Autodesk Inventor part; units mm, degrees
ref_plane "Work Plane1" through (0, 0, 1.25) normal (0, 0, 1) x (1, 0, 0)
ref_plane "YZ Plane" through (0, 0, 0) normal (1, 0, 0) x (0, 1, 0)
ref_plane "XZ Plane" through (0, 0, 0) normal (0, 1, 0) x (-1, 0, 0)
sketch "Sketch1" plane through (0, 0, 0) normal (0, 0, 1) x (1, 0, 0)
  circle A0 centre (0, 0) radius 5.5
  dimension "d0" = 11
extrude "Extrusion1" add sketch "Sketch1" along normal blind 2.5
hole "Hole1" at (0, 0, 2.5) direction (0, 0, -1) diameter 7 end through all
sketch "Sketch2" plane through (0, 0, 2.5) normal (0, 0, 1) x (1, 0, 0)
  circle A0 centre (0, 0) radius 5
  circle A1 centre (0, 0) radius 4
  dimension "d12" = 10
  dimension "d13" = 8
extrude "Extrusion2" cut sketch "Sketch2" against normal blind 0.5
ref_plane "Work Plane1" through (0, 0, 1.25) normal (0, 0, 1) x (1, 0, 0)
mirror "Mirror1" about plane through (0, 0, 1.25) normal (0, 0, 1) of "Extrusion2"
properties part number "bearing_7x11x2,5" material "Stainless Steel"
Build history of the part. All positions in model axes, mm. A direction names the side the tool comes from. Give positions to 0.01 mm unless a question says otherwise; leave off trailing zeros. Loops run counter-clockwise (first coordinate to the right, second up) from the corner with the lowest first, then second, coordinate; pieces in that order, holes last.
Item 1: Which spindle directions (+Z, -Z, +X, -X, +Y, -Y) get a long thin tool onto all of the face, cutting with end or side? Do faces 1 (the face through (1.341, -3.233, 1.232)), 2 (the face through (-0.867, -3.905, 2.254)), 3 (the face through (-0.867, 3.905, 0.246)). Say none if no direction does.
Answers follow:
face 1: +Z, -Z
face 2: +Z
face 3: -Z
Item 2: Slice it at A-A, the plane y = 0. List the corners of the cut face in (x, z), and give its area (3 significant figures).
Answers follow:
outline: (-5.5, 0) - (-5, 0) - (-5, 0.5) - (-4, 0.5) - (-4, 0) - (-3.5, 0) - (-3.5, 2.5) - (-4, 2.5) - (-4, 2) - (-5, 2) - (-5, 2.5) - (-5.5, 2.5) - close; (3.5, 0) - (4, 0) - (4, 0.5) - (5, 0.5) - (5, 0) - (5.5, 0) - (5.5, 2.5) - (5, 2.5) - (5, 2) - (4, 2) - (4, 2.5) - (3.5, 2.5) - close
area: 8.00 mm2
Item 3: Pull direction X, two halves, no side cores. Call faces 4 (the face through (1.6, -4.9, 0)), 5 (the face through (-1.08, -4.88, 2.25)), 6 (the face through (-1.19, 5.37, 1.23)), 7 (the face through (-1.08, 4.88, 0.25)): released by +X, released by -X, zero draft, split by the parting line, or undercut.
Answers follow:
face 4: zero draft
face 5: undercut
face 6: split by the parting line
face 7: undercut
Item 4: Slice it at B-B, the plane z = 0.2. List the corners of the cut face in (x, y), and give its area (3 significant figures).
Answers follow:
outline: circle Ø11 at (0, 0); circle Ø8 at (0, 0); hole circle Ø10 at (0, 0); hole circle Ø7 at (0, 0)
area: 28.3 mm2
Item 5: Slice it at D-D, the plane x = 4.75. List the corners of the cut face in (y, z).
Answers follow:
outline: (-2.77, 0) - (-1.56, 0) - (-1.56, 0.5) - (1.56, 0.5) - (1.56, 0) - (2.77, 0) - (2.77, 2.5) - (1.56, 2.5) - (1.56, 2) - (-1.56, 2) - (-1.56, 2.5) - (-2.77, 2.5) - close
Item 6: Flat gauge pins, fed straight in: pin 1 (2 mm diameter, centred on x = 2, y = 2.5, fed in from +Z); pin 2 (1 mm diameter, centred on y = 2, z = 1.5, fed in from -X). Where does each tip first touch, or does it go through?
Answers follow:
pin 1: stops at z = 2.5
pin 2: stops at x = -5.29
Item 7: Drill centre lines: line 1 (Y direction, x = 0, z = 1.1); line 2 (Y direction, x = -0.25, z = 0.25); line 3 (X direction, y = -1.5, z = 2.3). Where is each one in solid material? Low to high.
Answers follow:
line 1: y = -5.5 to -3.5, 3.5 to 5.5
line 2: y = -5.49 to -4.99, -3.99 to -3.49, 3.49 to 3.99, 4.99 to 5.49
line 3: x = -5.29 to -4.77, -3.71 to -3.16, 3.16 to 3.71, 4.77 to 5.29
Item 8: Slice it at C-C, the plane x = 2. List the corners of the cut face in (y, z), and give its area (3 significant figures).
Answers follow:
outline: (-5.12, 0) - (-4.58, 0) - (-4.58, 0.5) - (-3.46, 0.5) - (-3.46, 0) - (-2.87, 0) - (-2.87, 2.5) - (-3.46, 2.5) - (-3.46, 2) - (-4.58, 2) - (-4.58, 2.5) - (-5.12, 2.5) - close; (2.87, 0) - (3.46, 0) - (3.46, 0.5) - (4.58, 0.5) - (4.58, 0) - (5.12, 0) - (5.12, 2.5) - (4.58, 2.5) - (4.58, 2) - (3.46, 2) - (3.46, 2.5) - (2.87, 2.5) - close
area: 9.02 mm2
